Part model, mm, in its own coordinate system. A direction names the side the tool comes from. Round coordinates to 2 decimals unless told otherwise and drop trailing zeros. Order: outer loops, then holes, each group sorted by start corner. A loop starts at its lowest first (then second) coordinate and runs counter-clockwise, first axis right, second up. Notation, with made-up numbers: (37.25, 25) - (43.25, 25) arc R28 ccw to (43.25, 53) - close; hole circle Ø1 at (29, -24). An arc over 180 degrees is marked (long way). Return JSON: item names as keys, results as strings. Group by question number.
Item 1: Two-plate mould, pull along Y, no slides. Class faces 1 (the face through (-6, 0, 3)), 2 (the face through (7.723, -0.867, -3.905)), 3 (the face through (-8, 3, 3)): released by +Y, released by -Y, zero draft, split by the parting line, or undercut.
Item 2: Saw through at B-B on x = -1.75. List the corners of the cut face in (y, z), and give its area (3 significant figures).
Item 3: Saw through at A-A on x = 11.5. List the corners of the cut face in (y, z).
Item 4: Tool access for faces 4 (the face through (16, 0, 0)), 5 (the face through (0, 3, -3)), 6 (the face through (-6, -2.6, -1.5)): list every direction of +Z, -Z, +X, -X, +Y, -Y with a clear straight run to the whole face (end or side of a thin tool).
Item 5: Drop flat-ended pins along their axis: pin 1 (5 mm diameter, centred on x = 12.5, z = 1.5, fed in from -Y); pin 2 (6.5 mm diameter, centred on y = 3, z = -2, fed in from +X); pin 3 (1 mm diameter, centred on y = -1.5, z = -1, fed in from -X); pin 4 (4 mm diameter, centred on x = 11, y = 2.5, fed in from +Z). Give the stop position or say it passes through.
Item 6: Probe probe 1 along X at (y, z) = (3, -3.5); probe 2 along Z at (x, y) = (14.75, -2). List the from-to ranges inside material, lowest first.
Solid Edge part; units mm, degrees
sketch "Sketch1" plane through (0, 0, 0) normal (0, 0, 1) x (1, 0, 0)
  line L0 (-8, 0) -> (-8, 6)
  arc A0 (-8, 6) -> (-7.5, 6.5) centre (-7.5, 6) cw
  line L1 (-7.5, 6.5) -> (0, 6.5)
  line L2 (0, 6.5) -> (0, 4)
  line L3 (0, 4) -> (15.233, 4)
  line L4 (15.233, 4) -> (16, 3.233)
  line L5 (16, 3.233) -> (16, 0)
  line L6 (16, 0) -> (-8, 0)
revolve "RevolvedProtrusion1" add sketch "Sketch1" angle 360 about axis through (16, 0, 0) along (-1, 0, 0)
sketch "Sketch2" plane through (-8, 0, 0) normal (1, 0, 0) x (0, 1, 0)
  line L0 (-1.7321, 3) -> (-3.4641, 0)
  line L1 (-3.4641, 0) -> (-1.7321, -3)
  line L2 (-1.7321, -3) -> (1.7321, -3)
  line L3 (1.7321, -3) -> (3.4641, 0)
  line L4 (3.4641, 0) -> (1.7321, 3)
  line L5 (1.7321, 3) -> (-1.7321, 3)
extrude "ExtrudedCutout_1" cut sketch "Sketch2" along normal blind 4
sketch "Sketch3" plane through (0, 0, 0) normal (0, 0, 1) x (1, 0, 0)
  line L0 (-4, 0) -> (-4, 3)
  line L1 (-4, 3) -> (-2.1974, 0)
  line L2 (-2.1974, 0) -> (-4, 0)
revolve "RevolvedCutout1" cut sketch "Sketch3" angle 360 about axis through (-2.1974, 0, 0) along (-1, 0, 0)
cosmetic_thread "Rosca_3" thread depth 14
properties part number "07160-08X16"
Filled in:
{
 "1": {"face 1": "undercut", "face 2": "split by the parting line", "face 3": "zero draft"},
 "2": {"outline": "circle Ø13 at (0, 0)", "area": "133 mm^2"},
 "3": {"outline": "circle Ø8 at (0, 0)"},
 "4": {"face 4": "+Z, -Z, +X, +Y, -Y", "face 5": "+X", "face 6": "-X"},
 "5": {"pin 1": "stops at y = -4", "pin 2": "stops at x = 16", "pin 3": "stops at x = -3.58", "pin 4": "stops at z = 3.97"},
 "6": {"probe 1": "x = -8 to 0", "probe 2": "z = -3.46 to 3.46"}
}
